```python
from build123d import *

# Parameters (mm, degrees)
F0_R     = 63.946243
F0_R_2   = 5.334163
F1_DEPTH = 3.81


with BuildPart() as f1:
    # F0 (on Front) → F1 (new body)
    with BuildSketch(Plane.XZ):
        Circle(F0_R)
        with BuildLine():
            ThreePointArc((-0.355494, -28.829536), (-19.004092, -21.682089), (-28.534216, -4.131221))
            Line((-28.534216, -4.131221), (-9.421132, -4.131221))
            ThreePointArc((-9.421132, -4.131221), (-6.335532, -8.104675), (-1.734714, -10.139797))
            Line((-1.734714, -10.139797), (-0.355494, -28.829536))
        make_face(mode=Mode.SUBTRACT)
        with BuildLine():
            ThreePointArc((-57.030724, -4.131221), (-43.12199, 37.550825), (-3.747552, 57.05722))
            Line((-3.747552, 57.05722), (-3.747552, 31.774284))
            ThreePointArc((-3.747552, 31.774284), (-24.98442, 19.985696), (-31.821637, -3.321552))
            Line((-31.821637, -3.321552), (-35.653092, -4.131221))
            Line((-35.653092, -4.131221), (-31.726681, -4.131221))
            ThreePointArc((-31.726681, -4.131221), (-21.158247, -23.999539), (-0.121949, -31.994287))
            Line((-0.121949, -31.994287), (1.734714, -57.153839))
            ThreePointArc((1.734714, -57.153839), (-36.627394, -43.909048), (-56.53812, -8.544678))
            ThreePointArc((-56.53812, -8.544678), (-56.827284, -6.342733), (-57.030724, -4.131221))
        make_face(mode=Mode.SUBTRACT)
        with BuildLine():
            Line((-10.211481, 1.24514), (-28.70842, -2.663662))
            ThreePointArc((-28.70842, -2.663662), (-22.527775, 17.99355), (-3.747552, 28.587136))
            Line((-3.747552, 28.587136), (-3.747552, 9.580218))
            ThreePointArc((-3.747552, 9.580218), (-8.129086, 6.30418), (-10.211481, 1.24514))
        make_face(mode=Mode.SUBTRACT)
        Circle(F0_R_2, mode=Mode.SUBTRACT)
        with BuildLine():
            Line((0, 10.287114), (0, 28.831727))
            ThreePointArc((0, 28.831727), (18.420957, 22.179649), (28.341719, 5.292961))
            Line((28.341719, 5.292961), (9.193887, 4.614885))
            ThreePointArc((9.193887, 4.614885), (5.401429, 8.754958), (0, 10.287114))
        make_face(mode=Mode.SUBTRACT)
        with BuildLine():
            Line((0, 31.99452), (0, 57.180158))
            ThreePointArc((0, 57.180158), (38.724459, 42.071211), (56.984273, 4.728966))
            Line((56.984273, 4.728966), (30.757176, 8.811666))
            ThreePointArc((30.757176, 8.811666), (19.257781, 25.5497), (0, 31.99452))
        make_face(mode=Mode.SUBTRACT)
        with BuildLine():
            ThreePointArc((56.984273, 4.728966), (38.724459, 42.071211), (0, 57.180158))
            Line((0, 57.180158), (0, 31.99452))
            ThreePointArc((0, 31.99452), (19.257781, 25.5497), (30.757176, 8.811666))
            Line((30.757176, 8.811666), (56.984273, 4.728966))
        make_face()
    extrude(amount=F1_DEPTH)


solid = f1.part
```
Here's how the part is built. I have some questions about the finished solid (model axes, mm). A direction names the side the tool comes from. Give positions to 0.01 mm unless a question says otherwise; leave off trailing zeros. Order: outer loops, then holes, each group sorted by start corner. A loop starts at its lowest first (then second) coordinate and runs counter-clockwise, first axis right, second up. Notation, with made-up numbers: (-36, 63) -> (10, 63) arc R14 ccw to (10, 72) -> close; hole circle Ø9 at (66, 77.25). An arc over 180 degrees is marked (long way). Use CSV: the item, a comma, the result in double quotes. Start each with the question number.
Item 1: Suppose I cut it at A-A (y = -2.05). List the corners of the cut face in (x, z) for me, and give its area (3 significant figures).
Item 2: On a 3-axis mill with a long thin cutter (end or side, diameter ignored), from which of +Z, -Z, +X, -X, +Y, -Y can I reach the whole of each face in a straight line? I mean faces 1 (the flat face through (13, -3.81, 1)), 2 (the flat face through (-1.055, -1.878, -19.354)). Say none if no direction works.
Item 3: If I drill on probe 1 along X at (y, z) = (-2.85, 11.5); probe 2 along X at (y, z) = (-3.05, -8.5); probe 3 along Z at (x, y) = (4, -0.35), over which ranges is the centre line in solid material (lowest first)? Write a range as [from, to].
Item 4: I'm going to push flat-ended pins straight in: P1, Ø1.9, axis at y = -1.5, z = 21, coming from the -X side; P2, Ø1.9, axis at x = -16.5, y = -2, coming from the -Z side; P3, Ø2, axis at y = -3, z = 22.5, coming from the -X side; P4, Ø8, axis at x = -18.5, z = 10.5, coming from the +Y side. Where does each tip first touch, or does it pass through?
Item 5: Suppose I cut it at B-B (z = -38.5). List the corners of the cut face in (x, y) for me, and give its area (3 significant figures).
Item 6: Thinking about a two-plate mould opening in Z: for faces 3 (the flat face through (13, 0, 1)), 4 (the cylindrical face through (60.993, -1.878, 19.208)), 5 (the flat face through (-33.71, -1.88, -3.72)), which applies, pulls with the +Z half, pulls with the -Z half, needs draft (parallel to the pull), parting line crosses it, or undercut?
Item 7: Suppose I cut it at D-D (z = 13). List the corners of the cut face in (x, y) for me.
Item 8: Suppose I cut it at C-C (x = -43). List the corners of the cut face in (y, z) for me.
Answer block:
1,outline,"circle Ø127.89 at (0, 0); hole (-57.03, -4.13) arc R57.18 ccw to (-56.54, -8.54) arc R57.18 ccw to (1.73, -57.15) -> (-0.12, -31.99) arc R31.99 cw to (-31.73, -4.13) -> (-35.65, -4.13) -> (-31.82, -3.32) arc R31.99 cw to (-3.75, 31.77) -> (-3.75, 57.06) arc R57.18 ccw to start; hole (-28.71, -2.66) -> (-10.21, 1.25) arc R10.29 cw to (-3.75, 9.58) -> (-3.75, 28.59) arc R28.83 ccw to start; hole (-28.53, -4.13) arc R28.83 ccw to (-0.36, -28.83) -> (-1.73, -10.14) arc R10.29 cw to (-9.42, -4.13) -> close; hole circle Ø10.67 at (0, 0); hole (0, 10.29) arc R10.29 cw to (9.19, 4.61) -> (28.34, 5.29) arc R28.83 ccw to (0, 28.83) -> close"
1,area,"7,840 mm^2"
2,face 1,"+Z, -Z, +X, -X, -Y"
2,face 2,"+Y, -Y"
3,probe 1,"x = [-62.9, -56.01], [-29.86, -26.44], [-3.75, 0], [26.44, 62.9]"
3,probe 2,"x = [-63.38, -56.54], [-30.84, -27.55], [-5.79, 63.38]"
3,probe 3,"z = [-63.82, -3.53], [3.53, 9.48], [28.55, 63.82]"
4,P1,"stops at x = -60.72"
4,P2,"stops at z = -62.03"
4,P3,"stops at x = -60.22"
4,P4,"passes through"
5,outline,"(-51.06, -3.81) -> (-42.28, -3.81) -> (-42.28, 0) -> (-51.06, 0) -> close; (0.36, -3.81) -> (51.06, -3.81) -> (51.06, 0) -> (0.36, 0) -> close"
5,area,"227 mm^2"
6,face 3,"needs draft"
6,face 4,"parting line crosses it"
6,face 5,"undercut"
7,outline,"(-62.61, -3.81) -> (-55.68, -3.81) -> (-55.68, 0) -> (-62.61, 0) -> close; (-29.23, -3.81) -> (-25.73, -3.81) -> (-25.73, 0) -> (-29.23, 0) -> close; (-3.75, -3.81) -> (0, -3.81) -> (0, 0) -> (-3.75, 0) -> close; (25.73, -3.81) -> (62.61, -3.81) -> (62.61, 0) -> (25.73, 0) -> close"
8,outline,"(-3.81, -47.33) -> (0, -47.33) -> (0, -37.69) -> (-3.81, -37.69) -> close; (-3.81, 37.69) -> (0, 37.69) -> (0, 47.33) -> (-3.81, 47.33) -> close"
